Read the model definition and answer for the solid it produces. Units are mm, in the model's axes. Coordinates: 2 decimals unless noted, no trailing zeros. Write each loop counter-clockwise with the first axis right and the second up, starting at its lowest first coordinate (ties: lowest second). Pieces come first, ordered by that corner, then holes. Notation, with made-up numbers: M -14,-27.5 L -3,-27.5 A26 cw -3,-0.5 Z; hole C 21.5,50.5 d3. An arc over 180 degrees is marked long. Write item = value, one per line.
from build123d import *

# Parameters (mm, degrees)
SKETCH2_W             = 22
SKETCH2_H             = 17.825
SKETCH2_R             = 2.85
BOSS_EXTRUDE1_DEPTH   = 5.5
FILLET1_R             = 10
FILLET2_R             = 5.5
SKETCH4_R             = 2.55
CUT_EXTRUDE1_DEPTH    = 5.5
CHAMFER1_SIZE         = 0.4
CHAMFER1_SIZE2        = 1.098990968
CHAMFER4_SIZE         = 0.4
CHAMFER5_SIZE         = 0.4
CHAMFER5_SIZE2        = 1.098990968
BODY_MOVE_COPY1_ANGLE = 180
SKETCH5_W             = 35.5
SKETCH5_H             = 22
SKETCH5_R             = 1.6
SKETCH5_R_2           = 3.5
BOSS_EXTRUDE2_DEPTH   = 3.175
FILLET3_R             = 5.5


with BuildPart() as part:
    # Sketch2 → Boss-Extrude1 (new, symmetric)
    with BuildSketch(Plane(origin=(0, 0, 0), x_dir=(0, 0, -1), z_dir=(1, 0, 0))):
        with Locations((0, -2.0875)):
            Rectangle(SKETCH2_W, SKETCH2_H)
        Circle(SKETCH2_R, mode=Mode.SUBTRACT)
    extrude(amount=BOSS_EXTRUDE1_DEPTH, both=True)

    # Fillet1
    fillet1_edges = [part.edges().sort_by_distance(p)[0] for p in [
        (0, -11, -11),
        (0, -11, 11),
    ]]
    fillet(fillet1_edges, radius=FILLET1_R)

    # Fillet2
    fillet2_edges = [part.edges().sort_by_distance(p)[0] for p in [
        (-5.5, 2.9125, -11),
        (-5.5, -8.071067812, -8.071067812),
        (-5.5, -8.071067812, 8.071067812),
        (5.5, 2.9125, -11),
        (5.5, -8.071067812, -8.071067812),
        (5.5, -8.071067812, 8.071067812),
        (-5.5, 2.9125, 11),
        (5.5, 2.9125, 11),
        (-5.5, -11, 0),
        (5.5, -11, 0),
    ]]
    fillet(fillet2_edges, radius=FILLET2_R - 0.0001)  # a hair under: the kernel refuses the full size

    # Sketch4 → Cut-Extrude1 (cut)
    with BuildSketch(Plane(origin=(0, 6.825, 0), x_dir=(1, 0, 0), z_dir=(0, 1, 0))):
        with Locations(Location((0, 5.5, 0), (0, 0, 270))):
            Circle(SKETCH4_R)
        with Locations(Location((0, -5.5, 0), (0, 0, 270))):
            Circle(SKETCH4_R)
    extrude(amount=-CUT_EXTRUDE1_DEPTH, mode=Mode.SUBTRACT)

    # Chamfer1
    chamfer1_edges = [part.edges().sort_by_distance(p)[0] for p in [
        (-5.5, 0, 2.85),
    ]]
    chamfer1_side = [part.faces().sort_by_distance(p)[0] for p in [
        (-5.5, 6.659799367, 0),
    ]]
    chamfer(chamfer1_edges, length=CHAMFER1_SIZE, length2=CHAMFER1_SIZE2, reference=chamfer1_side[0])

    # Chamfer4
    chamfer4_edges = [part.edges().sort_by_distance(p)[0] for p in [
        (-5.5, 6.825, 0),
        (5.5, 6.825, 0),
        (3.889116586, 6.825, 9.389116586),
        (-3.889116586, 6.825, 9.389116586),
        (3.889116586, 6.825, -9.389116586),
        (-3.889116586, 6.825, -9.389116586),
    ]]
    chamfer(chamfer4_edges, length=CHAMFER4_SIZE)

    # Chamfer5
    chamfer5_edges = [part.edges().sort_by_distance(p)[0] for p in [
        (0, 6.825, -8.05),
        (0, 6.825, 2.95),
    ]]
    chamfer5_side = [part.faces().sort_by_distance(p)[0] for p in [
        (0, 6.825, 0),
    ]]
    chamfer(chamfer5_edges, length=CHAMFER5_SIZE, length2=CHAMFER5_SIZE2, reference=chamfer5_side[0])


with BuildPart() as body_2:
    # Body-Move/Copy1: copy of part
    add(part.part.rotate(Axis((0, 0, 0), (0, 1, 0)), BODY_MOVE_COPY1_ANGLE))


with BuildPart() as part_1:
    # Body-Move/Copy3: read off the stored shape, not the designer's step
    # Body-Move/Copy3: moved
    add(part.part.moved(Location((-24.5, 0, 0))))


with BuildPart() as body_3:
    # Sketch5 → Boss-Extrude2 (new body)
    with BuildSketch(Plane(origin=(0, 6.825, 0), x_dir=(1, 0, 0), z_dir=(0, 1, 0))):
        with Locations((-12.25, 0)):
            Rectangle(SKETCH5_W, SKETCH5_H)
        with Locations(Location((-24.5, 5.5, 0), (0, 0, 270))):
            Circle(SKETCH5_R, mode=Mode.SUBTRACT)
        with Locations(Location((0, -5.5, 0), (0, 0, 270))):
            Circle(SKETCH5_R, mode=Mode.SUBTRACT)
        with Locations(Location((0, 5.5, 0), (0, 0, 270))):
            Circle(SKETCH5_R, mode=Mode.SUBTRACT)
        with Locations(Location((-24.5, -5.5, 0), (0, 0, 270))):
            Circle(SKETCH5_R, mode=Mode.SUBTRACT)
        with Locations(Location((-12.25, 0, 0), (0, 0, 270))):
            Circle(SKETCH5_R_2, mode=Mode.SUBTRACT)
    extrude(amount=BOSS_EXTRUDE2_DEPTH)

    # Fillet3
    fillet3_edges = [body_3.edges().sort_by_distance(p)[0] for p in [
        (5.5, 8.4125, 11),
        (-30, 8.4125, 11),
        (-30, 8.4125, -11),
        (5.5, 8.4125, -11),
    ]]
    fillet(fillet3_edges, radius=FILLET3_R)


solid = body_3.part
Item 1: For a pull along X with two mould halves and no side action, classify faces 1 (the face through (-0.61, 8.39, -4.02)), 2 (the face through (5.5, 8, 0)), 3 (the face through (-8.6, 6.825, -0.2)) as released by +X, released by -X, zero draft, split by the parting line, or undercut.
Worked answers:
face_1 = undercut
face_2 = released by +X
face_3 = zero draft
Item 2: A flat-ended cylindrical pin translates along its axis: pin 1 (11 mm diameter, centred on x = -12.25, z = 0, fed in from +Y). Find the tip coordinate at first contact, or state that the pin passes through.
Worked answers:
pin_1 = 10
Item 3: Consider line 1 along X through (y, z) = (7.7, -5.5); line 2 along Z through (x, y) = (-23.5, 8.4); line 3 along Z through (x, y) = (-12.5, 7.75). Determine where each line is inside the solid, lowest interval first. Write a range as from..to.
Worked answers:
line_1 = -30..-26.1, -22.9..-1.6, 1.6..5.5
line_2 = -11..-6.75, -4.25..4.25, 6.75..11
line_3 = -11..-3.49, 3.49..11
Item 4: Find section A-A (y = 8.75). Determine the outline of the cut face in (x, z), and give its area (3 significant figures).
Worked answers:
outline = M -30,-5.5 A5.5 ccw -24.5,-11 L 0,-11 A5.5 ccw 5.5,-5.5 L 5.5,5.5 A5.5 ccw 0,11 L -24.5,11 A5.5 ccw -30,5.5 Z; hole C -24.5,-5.5 d3.2; hole C -24.5,5.5 d3.2; hole C -12.25,0 d7; hole C 0,-5.5 d3.2; hole C 0,5.5 d3.2
area = 684 mm²
Item 5: Find section C-C (z = 0). Determine the outline of the cut face in (x, y) (3 decimals).
Worked answers:
outline = M -30,6.825 L -15.75,6.825 L -15.75,10 L -30,10 Z; M -8.75,6.825 L 5.5,6.825 L 5.5,10 L -8.75,10 Z
Item 6: Find section B-B (x = -12.25). Determine the outline of the cut face in (y, z) (3 decimals).
Worked answers:
outline = M 6.825,-11 L 10,-11 L 10,-3.5 L 6.825,-3.5 Z; M 6.825,3.5 L 10,3.5 L 10,11 L 6.825,11 Z
